Source: CAD feature listing. Evaluate the final solid. Frame: model axes, mm. A direction names the side the tool comes from. Round coordinates to 2 decimals unless told otherwise and drop trailing zeros. Order: outer loops, then holes, each group sorted by start corner. A loop starts at its lowest first (then second) coordinate and runs counter-clockwise, first axis right, second up. Notation, with made-up numbers: M 48,30.25 L 63,30.25 A16 cw 63,53.25 Z; hole C 76,-30 d11. An arc over 180 degrees is marked long. Use one line per item in the form item = value. Start each with the question number.
Q1. Section D-D (y = 13.25). Return the cut outline in (x, z).
Q2. Reachability of faces 4 (the flat face through (1, 17, -13)), 5 (the flat face through (1, 13, -17)), 6 (the flat face through (3, 15, 13)) from +Z, -Z, +X, -X, +Y, -Y: full face, straight path, thin tool, end or side. Return the list, or none.
Q3. Pull-direction query (Z, two-part tool) for faces 1 (the flat face through (1, 13, 17)), 2 (the flat face through (10, 0, -17)), 3 (the cylindrical face through (9.86, 12.247, 0.269)); classes: pulls with the +Z half, pulls with the -Z half, needs draft (parallel to the pull), parting line crosses it, or undercut.
Q4. Section A-A (x = 16.5). Return the cut outline in (y, z), plus the area to 3 significant figures.
Q5. Section B-B (z = -18.75). Return the cut outline in (x, y), plus the area to 3 significant figures.
Q6. Section C-C (y = 2.5). Return the cut outline in (x, z).
Q7. Material intervals for probe 1 along X at (y, z) = (2.2, 18.75); probe 2 along Z at (x, y) = (16.5, 1.7); probe 3 along Z at (x, y) = (2.4, 15.5), sorted ascending.
Q8. Contact query for flat-ended pins moving along their axis: pin 1 (8 mm diameter, centred on x = 13, z = -18, fed in from +Y); pin 2 (1 mm diameter, centred on x = 2, y = 17, fed in from +Z); pin 3 (6.5 mm diameter, centred on y = 12, z = 16, fed in from +X). Output: stop coordinate, or through.
Autodesk Inventor part; units mm, degrees
ref_plane "YZ Plane" through (0, 0, 0) normal (1, 0, 0) x (0, 1, 0)
ref_plane "XZ Plane" through (0, 0, 0) normal (0, 1, 0) x (-1, 0, 0)
ref_plane "XY Plane" through (0, 0, 0) normal (0, 0, 1) x (1, 0, 0)
sketch "Skizze1" plane through (0, 0, 0) normal (1, 0, 0) x (0, 1, 0)
  arc A0 (0, -12.25) -> (0, 12.25) centre (0, 0) ccw
  arc A1 (0, -15.25) -> (0, 15.25) centre (0, 0) ccw
  line L0 (0, 15.25) -> (0, 12.25)
  line L1 (0, -12.25) -> (0, -15.25)
  dimension "d0" = 12.25
  dimension "d1" = 15.25
extrude "Extrusion1" add sketch "Skizze1" along normal blind 20
sketch "Skizze7" plane through (0, 0, 0) normal (-1, 0, 0) x (0, 0, 1)
  arc A0 (15.25, 0) -> (-15.25, 0) centre (0, 0) ccw
  line L0 (-12.5965, 8.596) -> (-21.1503, 17.1499)
  line L1 (-12.5965, 8.596) -> (-0.4995, 8.596) construction
  line L2 (-21.1503, 17.1499) -> (-17.1502, 21.15)
  line L3 (-17.1502, 21.15) -> (-8.596, 12.5965)
  arc A1 (-8.596, 12.5965) -> (-12.5965, 8.596) centre (0, 0) ccw
  dimension "d40" = 12.097
  dimension "d41" = 135
  dimension "d42" = 8.596
  dimension "d43" = 5.657
extrude "Extrusion4" add sketch "Skizze7" against normal blind 3
mirror "Spiegeln4" about plane through (0, 0, 0) normal (0, 0, 1) of "Extrusion4"
sketch "Skizze8" plane through (3, 21.15, 17.1502) normal (1, 0, 0) x (0, -0.7071, -0.7071)
  line L0 (-0.0002, -5.657) -> (0, 0)
  line L1 (29.9122, 24.2528) -> (24.2552, 24.253)
  line L2 (24.2552, 24.253) -> (24.2541, 12.156)
  line L3 (0, 0) -> (12.097, 0)
  point P0 (27.0822, -2.8294)
  point P1 (5.1619, -2.8285)
  point P2 (27.0832, 19.0909)
  point P3 (27.0837, 24.2529)
  dimension "d53" = 5.162
  dimension "d54" = 5.162
  dimension "d55" = 2.8285
  dimension "d56" = 2.8285
hole "Bohrung3" at (3, 15.5, 15.5001) at (3, 15.5, -15.5001) direction (-1, 0, 0) diameter 3.2 end through all
sketch "Skizze9" plane through (0, 0, 0) normal (-1, 0, 0) x (0, 0, 1)
  line L0 (-12.25, 0) -> (-15.25, 0)
  line L1 (-15.25, 0) -> (-22.25, 0)
  line L2 (-22.25, 0) -> (-22.25, 3)
  line L3 (-22.25, 3) -> (-14.952, 3)
  arc A0 (-12.5965, 8.596) -> (-15.25, 0) centre (0, 0) ccw
  arc A1 (-14.952, 3) -> (-15.25, 0) centre (0, 0) ccw
  dimension "d57" = 7
  dimension "d58" = 3
extrude "Extrusion5" add sketch "Skizze9" against normal blind 20
sketch "Skizze10" plane through (0, 0, -12.25) normal (0, -1, 0) x (1, 0, 0)
  line L0 (20, 0) -> (20, -10)
  line L1 (0, -10) -> (20, -10)
  point P0 (0, 12.25)
  point P1 (16.5, -6.5)
  dimension "d68" = 3.5
  dimension "d69" = 3.5
hole "Bohrung4" at (16.5, 0, -18.75) direction (0, 1, 0) diameter 3.2 end through all
mirror "Spiegeln5" about plane through (0, 0, 0) normal (0, 0, 1) of "Extrusion5", "Bohrung4"
properties part number "SensorHalterSchale"
Results list:
q1.outline = M 0,-17.25 L 3,-17.25 L 3,-9.25 L 0,-9.25 Z; M 0,-7.55 L 20,-7.55 L 20,7.55 L 0,7.55 Z; M 0,9.25 L 3,9.25 L 3,17.25 L 0,17.25 Z
q2.face_4 = +X, -X, +Y
q2.face_5 = -Z, +X, -X
q2.face_6 = +Z, +X, +Y
q3.face_1 = pulls with the +Z half
q3.face_2 = needs draft
q3.face_3 = undercut
q4.outline = M 0,-22.25 L 3,-22.25 L 3,-20.35 L 0,-20.35 Z; M 0,-17.15 L 3,-17.15 L 3,-14.95 A15.25 ccw 3,14.95 L 3,17.15 L 0,17.15 L 0,12.25 A12.25 cw 0,-12.25 Z; M 0,20.35 L 3,20.35 L 3,22.25 L 0,22.25 Z
q4.area = 153 mm2
q5.outline = M 0,0 L 14.9,0 L 14.9,3 L 0,3 Z; M 0,14.75 L 3,14.75 L 3,19.55 L 0,19.55 Z; M 18.1,0 L 20,0 L 20,3 L 18.1,3 Z
q5.area = 64.8 mm2
q6.outline = M 0,-22.25 L 20,-22.25 L 20,-11.99 L 0,-11.99 Z; M 0,11.99 L 20,11.99 L 20,22.25 L 0,22.25 Z; hole C 16.5,-18.75 d3.2; hole C 16.5,18.75 d3.2
q7.probe_1 = 0 to 14.9, 18.1 to 20
q7.probe_2 = -22.25 to -20.35, -17.15 to -12.13, 12.13 to 17.15, 20.35 to 22.25
q7.probe_3 = -19.5 to -17.1, -13.9 to -11.5, 11.5 to 13.9, 17.1 to 19.5
q8.pin_1 = 6.05
q8.pin_2 = 21.15
q8.pin_3 = 3
